Can you work these out from the model? Positions are in its coordinate system, mm. Coordinates: 2 decimals unless noted, no trailing zeros. Loops run counter-clockwise (first coordinate to the right, second up) from the corner with the lowest first, then second, coordinate; pieces in that order, holes last.
```python
from build123d import *

# Parameters (mm, degrees)
F1_DEPTH = 3


with BuildPart() as f1:
    # F0 (on Front) → F1 (new body)
    with BuildSketch(Plane.XZ):
        Polygon((7.4, -3), (0, -3), (0, -6), (3, -6), (3, -9.6), (0, -9.6), (0, -12.6), (7.4, -12.6), (7.4, -15.6), (13.7, -15.6), (13.7, -12.6), (20, -12.6), (20, -15.6), (26.3, -15.6), (26.3, -12.6), (32.6, -12.6), (32.6, -15.6), (42, -15.6), (42, -12.6), (48.3, -12.6), (48.3, -15.6), (54.6, -15.6), (54.6, -12.6), (60.9, -12.6), (60.9, -15.6), (67.2, -15.6), (67.2, -12.6), (74.6, -12.6), (74.6, -9.6), (71.6, -9.6), (71.6, -6), (74.6, -6), (74.6, 0), (29.3, 0), (29.3, -3), (26.3, -3), (26.3, 0), (20, 0), (20, -3), (13.7, -3), (13.7, 0), (7.4, 0), align=None)
    extrude(amount=-F1_DEPTH)


solid = f1.part
```
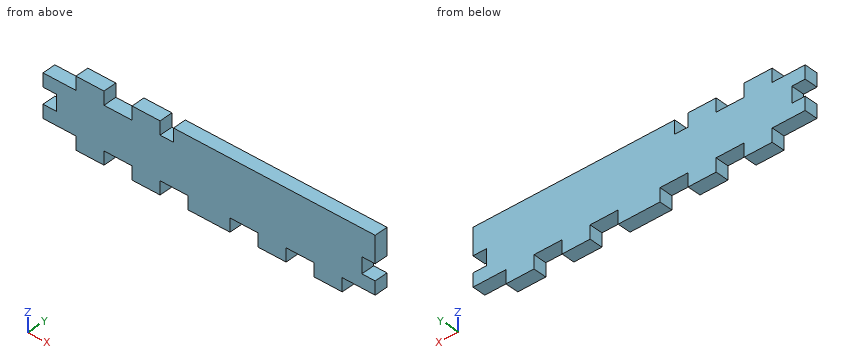
(1) I want a section at B-B on x = 31.5. Write out the boundary of the cut face in (y, z).
Check values:
outline: (0, -12.6) - (3, -12.6) - (3, 0) - (0, 0) - close
(2) If I drill on probe 1 along X at (y, z) = (2.15, -2.75); probe 2 along X at (y, z) = (2.4, -13.25); probe 3 along X at (y, z) = (2.7, -6.75), over which ranges is the centre line in solid material (lowest first)?
Check values:
probe 1: x = 7.4 to 13.7, 20 to 26.3, 29.3 to 74.6
probe 2: x = 7.4 to 13.7, 20 to 26.3, 32.6 to 42, 48.3 to 54.6, 60.9 to 67.2
probe 3: x = 3 to 71.6
(3) I'm going to push flat-ended pins straight in: pin 1 (0.9 mm diameter, centred on y = 1.5, z = -14.5, fed in from -X); pin 2 (0.9 mm diameter, centred on x = 45, y = 1, fed in from -Z); pin 3 (0.9 mm diameter, centred on y = 2, z = -14, fed in from +X). Where does each tip first touch, or does it pass through?
Check values:
pin 1: stops at x = 7.4
pin 2: stops at z = -12.6
pin 3: stops at x = 67.2
(4) I want a section at C-C on z = -8.25. Write out the boundary of the cut face in (x, y), then the cut area to 3 significant figures.
Check values:
outline: (3, 0) - (71.6, 0) - (71.6, 3) - (3, 3) - close
area: 206 mm2
(5) I want a section at A-A on z = -0.75. Write out the boundary of the cut face in (x, y), then the cut area to 3 significant figures.
Check values:
outline: (7.4, 0) - (13.7, 0) - (13.7, 3) - (7.4, 3) - close; (20, 0) - (26.3, 0) - (26.3, 3) - (20, 3) - close; (29.3, 0) - (74.6, 0) - (74.6, 3) - (29.3, 3) - close
area: 174 mm2
